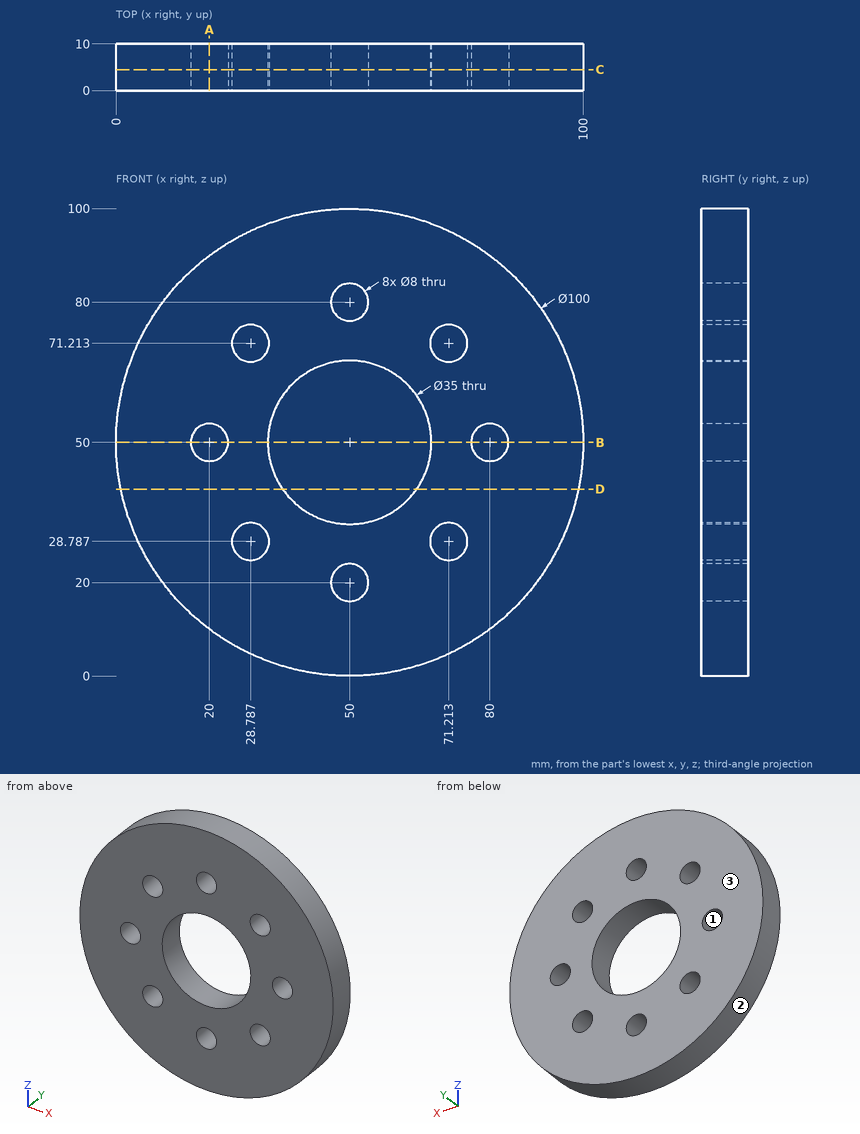
Can you work these out from the drawing? Everything is in mm from the part's minimum corner. Coordinates: 2 decimals unless noted, no trailing zeros. Loops run counter-clockwise (first coordinate to the right, second up) from the corner with the lowest first, then second, coordinate; pieces in that order, holes last. Notation, with made-up numbers: (0, 2.5) - (41, 2.5) arc R29 cw to (41, 23.5) - close; hole circle Ø10 at (45, 84). An arc over 180 degrees is marked (long way). Put each result on its own line as item: value. Start each with the question number.
Item 1: Suppose I cut it at A-A (x = 20). Please give me the cut outline in (y, z).
Item 2: If I drill on line 1 along Z through (x, y) = (50, 6.5); line 2 along X through (y, z) = (4.5, 30) (1 decimal); line 3 along X through (y, z) = (7.75, 39) (1 decimal), over which ranges is the centre line in solid material (lowest first)?
Item 3: Suppose I cut it at C-C (y = 4.5). State how many separate pieces and enclosed holes the cut face has, and give its area (3 significant figures).
Item 4: For pin 1 (4 mm diameter, centred on y = 1.5, z = 66, fed in from -X); pin 2 (2 mm diameter, centred on x = 88, y = 6, fed in from -Z); pin 3 (5 mm diameter, centred on x = 31, y = 7.5, fed in from +Z), each with a flat end and sliding along its axis, tell me the tip position at first contact or that it passes through.
Item 5: Suppose I cut it at B-B (z = 50). Please give me the cut outline in (x, y).
Item 6: Suppose I cut it at D-D (z = 40). Please give me the cut outline in (x, y).
Item 7: If we mould it in two halves opening along X, with no side actions, what happens to the marked faces 1, 2 and 3? For each: +X half, -X half, draft (parallel to the pull), parting line (faces both ways), or undercut.
Here are the results:
1. outline: (0, 10) - (10, 10) - (10, 46) - (0, 46) - close; (0, 54) - (10, 54) - (10, 90) - (0, 90) - close
2. line 1: 0 to 16, 24 to 32.5, 67.5 to 76, 84 to 100
2. line 2: 4.2 to 25, 32.6 to 67.4, 75 to 95.8
2. line 3: 1.2 to 36.4, 63.6 to 98.8
3. separate pieces: 1
3. enclosed holes: 9
3. area: 6,490 mm²
4. pin 1: x = 2
4. pin 2: z = 16.37
4. pin 3: z = 97.2
5. outline: (0, 0) - (16, 0) - (16, 10) - (0, 10) - close; (24, 0) - (32.5, 0) - (32.5, 10) - (24, 10) - close; (67.5, 0) - (76, 0) - (76, 10) - (67.5, 10) - close; (84, 0) - (100, 0) - (100, 10) - (84, 10) - close
6. outline: (1.01, 0) - (35.64, 0) - (35.64, 10) - (1.01, 10) - close; (64.36, 0) - (98.99, 0) - (98.99, 10) - (64.36, 10) - close
7. face 1: undercut
7. face 2: parting line
7. face 3: draft
